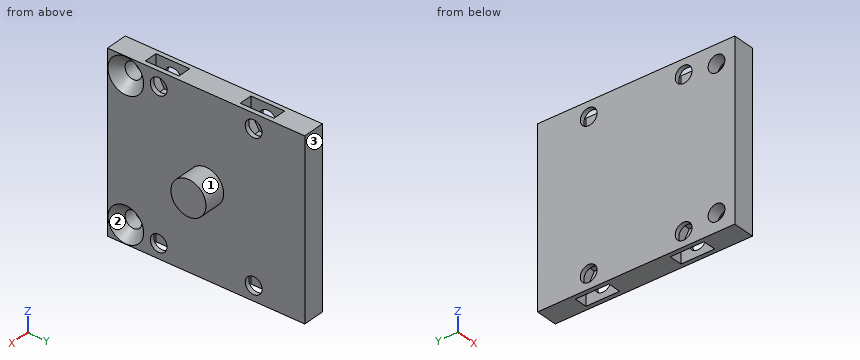
from build123d import *

# Parameters (mm, degrees)
SKETCH1_W           = 24
SKETCH1_H           = 27
SKETCH1_R           = 1.15
BOSS_EXTRUDE1_DEPTH = 3
SKETCH2_R           = 2.4
BOSS_EXTRUDE2_DEPTH = 3
CHAMFER1_SIZE       = 1.3
SKETCH3_R           = 1.15
CUT_EXTRUDE1_DEPTH  = 3
CUT_EXTRUDE2_START  = 0.6
CUT_EXTRUDE2_DEPTH  = 1.8
SKETCH5_W           = 2
SKETCH5_H           = 4.618802154
CUT_EXTRUDE3_DEPTH  = 1.8


with BuildPart() as part:
    # Sketch1 → Boss-Extrude1 (new body)
    with BuildSketch(Plane(origin=(0, 0, 0), x_dir=(0, 0, -1), z_dir=(1, 0, 0))):
        Rectangle(SKETCH1_W, SKETCH1_H)
        with Locations((-9.5, -11)):
            Circle(SKETCH1_R, mode=Mode.SUBTRACT)
        with Locations((9.5, -11)):
            Circle(SKETCH1_R, mode=Mode.SUBTRACT)
    extrude(amount=BOSS_EXTRUDE1_DEPTH)

    # Sketch2 → Boss-Extrude2 (add)
    with BuildSketch(Plane(origin=(3, 0, 0), x_dir=(0, 0, -1), z_dir=(1, 0, 0))):
        Circle(SKETCH2_R)
    extrude(amount=BOSS_EXTRUDE2_DEPTH)

    # Chamfer1
    chamfer1_edges = [part.edges().sort_by_distance(p)[0] for p in [
        (3, -11, 10.65),
        (3, -11, -8.35),
    ]]
    chamfer(chamfer1_edges, length=CHAMFER1_SIZE)

    # Sketch3 → Cut-Extrude1 (cut)
    with BuildSketch(Plane(origin=(0, 0, 0), x_dir=(0, 0, -1), z_dir=(1, 0, 0))):
        with Locations((-10, 6.5)):
            Circle(SKETCH3_R)
        with Locations((-10, -6.5)):
            Circle(SKETCH3_R)
        with Locations((10, -6.5)):
            Circle(SKETCH3_R)
        with Locations((10, 6.5)):
            Circle(SKETCH3_R)
    extrude(amount=CUT_EXTRUDE1_DEPTH, mode=Mode.SUBTRACT)

    # Sketch4 → Cut-Extrude2 (cut)
    with BuildSketch(Plane(origin=(0, 0, 0), x_dir=(0, 0, -1), z_dir=(1, 0, 0)).offset(CUT_EXTRUDE2_START)):
        Polygon((-10, 4.190598923), (-8, 5.345299462), (-8, 7.654700538), (-10, 8.809401077), (-12, 7.654700538), (-12, 5.345299462), align=None)
        Polygon((-10, -4.190598923), (-12, -5.345299462), (-12, -7.654700538), (-10, -8.809401077), (-8, -7.654700538), (-8, -5.345299462), align=None)
        Polygon((10, -4.190598923), (8, -5.345299462), (8, -7.654700538), (10, -8.809401077), (12, -7.654700538), (12, -5.345299462), align=None)
        Polygon((10, 8.809401077), (8, 7.654700538), (8, 5.345299462), (10, 4.190598923), (12, 5.345299462), (12, 7.654700538), align=None)
    extrude(amount=CUT_EXTRUDE2_DEPTH, mode=Mode.SUBTRACT)

    # Sketch5 → Cut-Extrude3 (cut)
    with BuildSketch(Plane(origin=(0.6, 0, 0), x_dir=(0, 0, -1), z_dir=(1, 0, 0))):
        with Locations((-11, 6.5)):
            Rectangle(SKETCH5_W, SKETCH5_H)
        with Locations((-11, -6.5)):
            Rectangle(SKETCH5_W, SKETCH5_H)
        with Locations((11, 6.5)):
            Rectangle(SKETCH5_W, SKETCH5_H)
        with Locations((11, -6.5)):
            Rectangle(SKETCH5_W, SKETCH5_H)
    extrude(amount=CUT_EXTRUDE3_DEPTH, mode=Mode.SUBTRACT)


solid = part.part
Geometry: final body of the model. Coordinates: model frame, mm. Face numbers are marked on the shaded views. Coordinates: 2 decimals unless noted, no trailing zeros. Order: outer loops, then holes, each group sorted by start corner. A loop starts at its lowest first (then second) coordinate and runs counter-clockwise, first axis right, second up.
(1) Draft query along Z for the marked faces 1, 2 and 3. Return one class per face: pulls with the +Z half, pulls with the -Z half, needs draft (parallel to the pull), parting line crosses it, or undercut.
(2) Section query A-A (y = 6.5). Return the cut outline in (x, z).
(3) Material intervals for probe 1 along Z at (x, y) = (2.7, -6.5); probe 2 along Y at (x, z) = (1.2, 10.75); probe 3 along Y at (x, z) = (1.4, -9.75), sorted ascending.
(4) First-contact query: pin 1 (4.5 mm diameter, centred on y = 7.5, z = 11, fed in from +X); pin 2 (0.5 mm diameter, centred on x = 1, y = 7, fed in from -Z); pin 3 (3.5 mm diameter, centred on y = -11, z = -9.5, fed in from +X). Flat tips, straight axial feed; report the tip coordinate or a pass-through.
(5) Section query B-B (x = 2.1). State how many separate pieces and enclosed holes the cut face has, plus the area to 3 significant figures.
(6) Section query C-C (y = -11). Return the cut outline in (x, z), plus the area to 3 significant figures.
Solution:
1. face 1: parting line crosses it
1. face 2: undercut
1. face 3: needs draft
2. outline: (0, -12) - (0.6, -12) - (0.6, -11.15) - (0, -11.15) - close; (0, -8.85) - (0.6, -8.85) - (0.6, -8) - (2.4, -8) - (2.4, -8.85) - (3, -8.85) - (3, 8.85) - (2.4, 8.85) - (2.4, 8) - (0.6, 8) - (0.6, 8.85) - (0, 8.85) - close; (0, 11.15) - (0.6, 11.15) - (0.6, 12) - (0, 12) - close; (2.4, -12) - (3, -12) - (3, -11.15) - (2.4, -11.15) - close; (2.4, 11.15) - (3, 11.15) - (3, 12) - (2.4, 12) - close
3. probe 1: z = -12 to -11.15, -8.85 to 8.85, 11.15 to 12
3. probe 2: y = -13.5 to -8.81, -4.19 to 4.19, 8.81 to 13.5
3. probe 3: y = -13.5 to -12.12, -9.88 to -8.67, -4.33 to 4.33, 8.67 to 13.5
4. pin 1: stops at x = 3
4. pin 2: stops at z = -8
4. pin 3: stops at x = 2.3
5. separate pieces: 1
5. enclosed holes: 2
5. area: 568 mm2
6. outline: (0, -12) - (3, -12) - (3, -11.95) - (1.7, -10.65) - (0, -10.65) - close; (0, -8.35) - (1.7, -8.35) - (3, -7.05) - (3, 7.05) - (1.7, 8.35) - (0, 8.35) - close; (0, 10.65) - (1.7, 10.65) - (3, 11.95) - (3, 12) - (0, 12) - close
6. area: 54.8 mm2
